Drawing for the job (mm, zero at the part's lowest x, y, z). Coordinates: 2 decimals unless noted, no trailing zeros. Loops run counter-clockwise (first coordinate to the right, second up) from the corner with the lowest first, then second, coordinate; pieces in that order, holes last. Notation, with made-up numbers: (-16.75, 61.5) - (5.25, 61.5) arc R6 cw to (5.25, 66.5) - close; hole circle Ø5 at (87.25, 46). An arc over 180 degrees is marked (long way). Put each result on its own line as item: value.
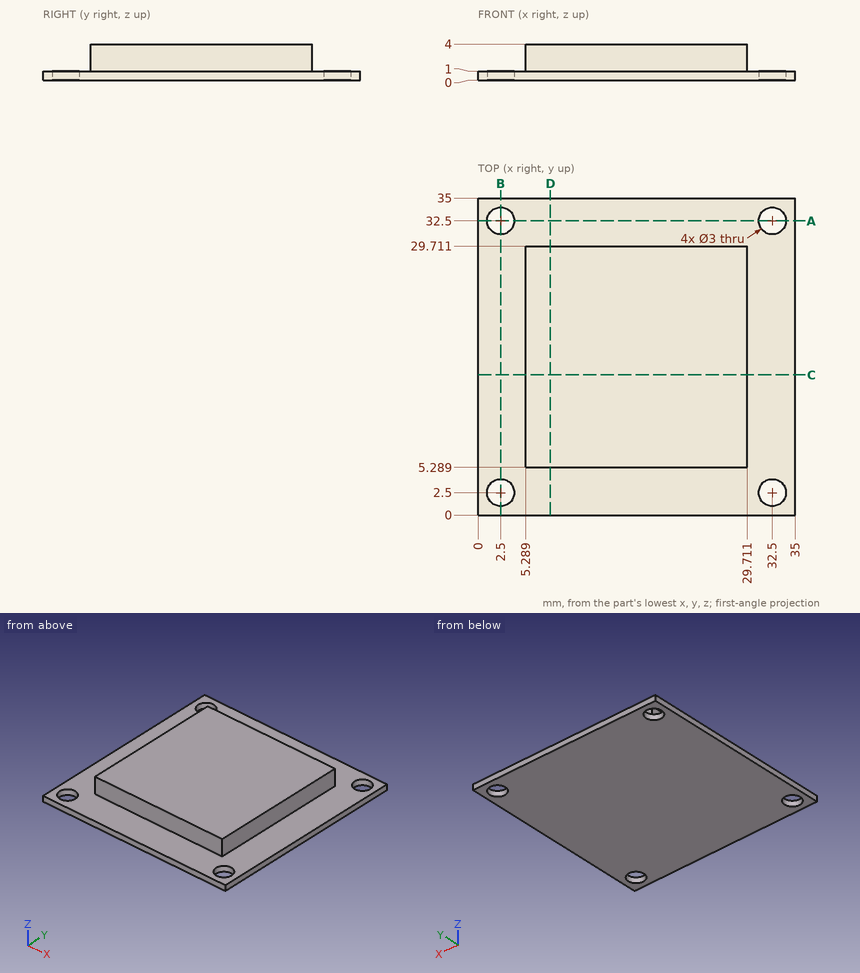
Q1. Wall check: L1, parallel to Y at x = 32.5, z = 0.25; L2, parallel to Z at x = 5, y = 18; L3, parallel to Y at x = 6, z = 2.35. Give the ranges that are in metal, low to high. Write a range as from..to.
Determined:
L1: 0..1, 4..31, 34..35
L2: 0..1
L3: 5.29..29.71
Q2. Slice it at A-A, the plane y = 32.5. Give the cut face in (x, z).
Determined:
outline: (0, 0) - (1, 0) - (1, 1) - (0, 1) - close; (4, 0) - (31, 0) - (31, 1) - (4, 1) - close; (34, 0) - (35, 0) - (35, 1) - (34, 1) - close
Q3. Pin check, flat tips, straight feed: pin 1 Ø2.5 at (x, y) = (2.5, 32.5) entering from +Z; pin 2 Ø0.9 at (y, z) = (14, 2) entering from +X; pin 3 Ø4 at (x, y) = (2.5, 2.5) entering from +Z. Stop position of each tip, or through.
Determined:
pin 1: through
pin 2: x = 29.71
pin 3: z = 1
Q4. Slice it at C-C, the plane y = 15.5. Give the cut face in (x, z).
Determined:
outline: (0, 0) - (35, 0) - (35, 1) - (29.71, 1) - (29.71, 4) - (5.29, 4) - (5.29, 1) - (0, 1) - close
